```python
from build123d import *

# Parameters (mm, degrees)
RESSALTO_EXTRUS_O1_DEPTH = 2
CORTE_EXTRUS_O1_REACH    = 58.091
ESBO_O2_R                = 0.85
RESSALTO_EXTRUS_O2_START = 1.9
ESBO_O4_R                = 2.5
RESSALTO_EXTRUS_O2_DEPTH = 1.9
CORTE_EXTRUS_O2_REACH    = 58.191
ESBO_O3_R                = 0.5


with BuildPart() as part:
    # Esboço1 → Ressalto-extrusão1 (new body)
    with BuildSketch(Plane(origin=(0, 0, 0), x_dir=(0, 0, -1), z_dir=(1, 0, 0))):
        with BuildLine():
            Line((0, 2.5), (53.5, 2.5))
            ThreePointArc((53.5, 2.5), (56, 0), (53.5, -2.5))
            Line((53.5, -2.5), (0, -2.5))
            ThreePointArc((0, -2.5), (-2.5, 0), (0, 2.5))
        make_face()
    extrude(amount=RESSALTO_EXTRUS_O1_DEPTH)

    # Esboço2 → Corte-extrusão1 (cut, up to next)
    with BuildSketch(Plane(origin=(2, 0, 0), x_dir=(0, 0, -1), z_dir=(1, 0, 0)), mode=Mode.PRIVATE) as corte_extrus_o1_sk1:
        Circle(ESBO_O2_R)
    corte_extrus_o1_tool1 = extrude(corte_extrus_o1_sk1.sketch, amount=-CORTE_EXTRUS_O1_REACH, mode=Mode.PRIVATE) & part.part
    add(corte_extrus_o1_tool1.solids().sort_by_distance((2, 0, 0))[0], mode=Mode.SUBTRACT)

    # Esboço4 → Ressalto-extrusão2 (add)
    with BuildSketch(Plane.ZY.offset(RESSALTO_EXTRUS_O2_START)):
        with Locations((-53.5, 0)):
            Circle(ESBO_O4_R)
    extrude(amount=-RESSALTO_EXTRUS_O2_DEPTH)

    # Esboço3 → Corte-extrusão2 (cut, up to next)
    with BuildSketch(Plane(origin=(2, 0, 0), x_dir=(0, 0, -1), z_dir=(1, 0, 0)), mode=Mode.PRIVATE) as corte_extrus_o2_sk1:
        with Locations((53.5, 0)):
            Circle(ESBO_O3_R)
    corte_extrus_o2_tool1 = extrude(corte_extrus_o2_sk1.sketch, amount=-CORTE_EXTRUS_O2_REACH, mode=Mode.PRIVATE) & part.part
    add(corte_extrus_o2_tool1.solids().sort_by_distance((2, 0, -53.5))[0], mode=Mode.SUBTRACT)


solid = part.part
```
Build history of the part. All positions in model axes, mm. A direction names the side the tool comes from. Round coordinates to 2 decimals unless told otherwise and drop trailing zeros. Order: outer loops, then holes, each group sorted by start corner. A loop starts at its lowest first (then second) coordinate and runs counter-clockwise, first axis right, second up. Notation, with made-up numbers: (60, 0.25) -> (105, 0.25) arc R23 cw to (105, 31.25) -> close; hole circle Ø2 at (27, -10.75). An arc over 180 degrees is marked (long way). Answer in a Markdown table with one row per item.
1) Mould opens along Y. For faces 1 (the cylindrical face through (0, 0, -53)), 2 (the flat face through (1, 2.5, -26)), 3 (the flat face through (-1.9, -1, -54)) say: released by +Y, released by -Y, zero draft, split by the parting line, or undercut.
Values:
| item | result |
|---|---|
| face 1 | undercut |
| face 2 | released by +Y |
| face 3 | zero draft |
2) Pin check, flat tip, straight feed: P1, Ø1.5, axis at y = 0, z = -21.5, coming from the -X side. Stop position of the tip, or through.
Values:
| item | result |
|---|---|
| P1 | x = 0 |
3) Band-saw the part on A-A on y = 0. Give the cut face in (x, z).
Values:
| item | result |
|---|---|
| outline | (-1.9, -56) -> (2, -56) -> (2, -54) -> (-1.9, -54) -> close; (-1.9, -53) -> (2, -53) -> (2, -0.85) -> (0, -0.85) -> (0, -51) -> (-1.9, -51) -> close; (0, 0.85) -> (2, 0.85) -> (2, 2.5) -> (0, 2.5) -> close |
4) Band-saw the part on C-C on z = -32. Give the cut face in (x, y), and give its area (3 significant figures).
Values:
| item | result |
|---|---|
| outline | (0, -2.5) -> (2, -2.5) -> (2, 2.5) -> (0, 2.5) -> close |
| area | 10.0 mm2 |
5) Which spindle directions (+Z, -Z, +X, -X, +Y, -Y) get a long thin tool onto all of the face, cutting with end or side? Do faces 4 (the cylindrical face through (1.01, -0.83, 0.18)), 5 (the cylindrical face through (0, 0, -56)). Say none if no direction does.
Values:
| item | result |
|---|---|
| face 4 | +X, -X |
| face 5 | -X |
6) Wall check: L1, parallel to Y at x = -0.4, z = -53.5; L2, parallel to X at y = 1.65, z = -24.5; L3, parallel to Z at x = 1.7, y = -0.75. Give the ranges that are in metal, low to high.
Values:
| item | result |
|---|---|
| L1 | -2.5 to -0.5, 0.5 to 2.5 |
| L2 | 0 to 2 |
| L3 | -55.88 to -0.4, 0.4 to 2.38 |
7) Band-saw the part on B-B on x = 1.1. Give the cut face in (y, z), and give its area (3 significant figures).
Values:
| item | result |
|---|---|
| outline | (-2.5, -53.5) arc R2.5 ccw to (2.5, -53.5) -> (2.5, 0) arc R2.5 ccw to (-2.5, 0) -> close; hole circle Ø1.7 at (0, 0); hole circle Ø1 at (0, -53.5) |
| area | 284 mm2 |
